from build123d import *

# Parameters (mm, degrees)
SKETCH1_R           = 7.5
BOSS_EXTRUDE2_DEPTH = 5
BOSS_EXTRUDE5_START = 2.5
SKETCH4_R           = 5
BOSS_EXTRUDE5_DEPTH = 5
BOSS_EXTRUDE6_START = -7.5
SKETCH4_2_R         = 5
BOSS_EXTRUDE6_DEPTH = 5
CIRPATTERN5_COUNT   = 3
CIRPATTERN5_ANGLE   = 240


with BuildPart() as part:
    # Sketch1 → Boss-Extrude2 (new body)
    with BuildSketch(Plane(origin=(0, 0, 0), x_dir=(1, 0, 0), z_dir=(0, 1, 0))):
        with BuildLine():
            Line((-15, 98.868599666), (-15, 128.868599666))
            Line((-15, 128.868599666), (15, 128.868599666))
            Line((15, 128.868599666), (15, 98.868599666))
            ThreePointArc((15, 98.868599666), (86.602540378, 50), (93.122718948, -36.443918776))
            Line((93.122718948, -36.443918776), (119.103481061, -51.443918776))
            Line((119.103481061, -51.443918776), (104.103481061, -77.42468089))
            Line((104.103481061, -77.42468089), (78.122718948, -62.42468089))
            ThreePointArc((78.122718948, -62.42468089), (0, -100), (-78.122718948, -62.42468089))
            Line((-78.122718948, -62.42468089), (-104.103481061, -77.42468089))
            Line((-104.103481061, -77.42468089), (-119.103481061, -51.443918776))
            Line((-119.103481061, -51.443918776), (-93.122718948, -36.443918776))
            ThreePointArc((-93.122718948, -36.443918776), (-86.602540378, 50), (-15, 98.868599666))
        make_face()
        with Locations(Location((0, 0, 0), (0, 0, 270))):
            Circle(SKETCH1_R, mode=Mode.SUBTRACT)
    extrude(amount=BOSS_EXTRUDE2_DEPTH)

    # Sketch4 → Boss-Extrude5 (add)
    with BuildSketch(Plane(origin=(0, 0, 0), x_dir=(0, 0, -1), z_dir=(1, 0, 0)).offset(BOSS_EXTRUDE5_START)):
        with BuildLine():
            Line((104.299170688, -17.902762311), (98.868599666, 0))
            Line((98.868599666, 0), (128.868599666, 0))
            Line((128.868599666, 0), (123.438028644, -17.902762311))
            ThreePointArc((123.438028644, -17.902762311), (113.868599666, -25), (104.299170688, -17.902762311))
        make_face()
        with Locations((113.868599666, -15)):
            Circle(SKETCH4_R, mode=Mode.SUBTRACT)
    boss_extrude5 = extrude(amount=BOSS_EXTRUDE5_DEPTH)

    # Sketch4_2 → Boss-Extrude6 (add)
    with BuildSketch(Plane(origin=(0, 0, 0), x_dir=(0, 0, -1), z_dir=(1, 0, 0)).offset(BOSS_EXTRUDE6_START)):
        with BuildLine():
            Line((104.299170688, -17.902762311), (98.868599666, 0))
            Line((98.868599666, 0), (128.868599666, 0))
            Line((128.868599666, 0), (123.438028644, -17.902762311))
            ThreePointArc((123.438028644, -17.902762311), (113.868599666, -25), (104.299170688, -17.902762311))
        make_face()
        with Locations((113.868599666, -15)):
            Circle(SKETCH4_2_R, mode=Mode.SUBTRACT)
    boss_extrude6 = extrude(amount=BOSS_EXTRUDE6_DEPTH)

    # CirPattern5: Boss-Extrude5, Boss-Extrude6 ×3 about axis
    cirpattern5_axis = Axis((0, 0, 0), (0, 1, 0))
    add([boss_extrude5.rotate(cirpattern5_axis, i * CIRPATTERN5_ANGLE / (CIRPATTERN5_COUNT - 1)) for i in range(1, CIRPATTERN5_COUNT)])
    add([boss_extrude6.rotate(cirpattern5_axis, i * CIRPATTERN5_ANGLE / (CIRPATTERN5_COUNT - 1)) for i in range(1, CIRPATTERN5_COUNT)])


solid = part.part
Design review of the part built by this model. Coordinates are the model's own, in mm. A direction names the side the tool comes from. Give positions to 0.01 mm unless a question says otherwise; leave off trailing zeros. Order: outer loops, then holes, each group sorted by start corner. A loop starts at its lowest first (then second) coordinate and runs counter-clockwise, first axis right, second up. Notation, with made-up numbers: (25.25, 55) - (52.25, 55) arc R29 ccw to (52.25, 80) - close; hole circle Ø10 at (-27.5, 83). An arc over 180 degrees is marked (long way). Write item = value, one per line. Start each with the question number.
Q1. Tool access review of faces 5 (the face through (102.54, -9.55, 50.54)), 6 (the face through (-7.5, -9.5, -114.1)), 7 (the face through (-106.295, 2.465, 44.049)), 8 (the face through (-95.04, -9.55, 63.53)): name each direction out of +Z, -Z, +X, -X, +Y, -Y from which nothing blocks a thin tool from reaching the whole face with its end or side.
Q2. We need section B-B on y = -3.75. State the section outline as (x, z) points, plus the area to 3 significant figures.
Q3. We need section C-C on x = 28. State the section outline as (y, z) points.
Q4. To check wall thickness, follow L1, parallel to X at y = 2.3, z = 0; L2, parallel to X at y = -7.25, z = -115.5; L3, parallel to X at y = 0.5, z = -100. State the ranges of each line that lie inside material, in increasing order. Write a range as from..to.
Q5. Clearance check with flat-ended pins moving along their axes: pin 1 Ø5.5 at (y, z) = (1.5, -116) entering from -X; pin 2 Ø12.5 at (y, z) = (-7.5, -121) entering from +X; pin 3 Ø11.5 at (y, z) = (-15, -113.87) entering from -X. State where each tip first meets the part, or that it passes through.
Q6. We need section D-D on z = -39. State the section outline as (x, y) points.
Q7. We need section A-A on z = 0. State the section outline as (x, y) points.
Q8. Mouldability with a two-part tool opening along Z and no side actions: class faces 1 (the face through (0.33, 2.465, -7.493)), 2 (the face through (105.13, -16.92, 54.88)), 3 (the face through (-5, -25, -114)), 4 (the face through (106.8, -8.83, 67.4)) as released by +Z, released by -Z, zero draft, split by the parting line, or undercut.
Working result:
q1.face_5 = -Z, +X, -Y
q1.face_6 = +Z, -Z, -X, -Y
q1.face_7 = -X, +Y, -Y
q1.face_8 = +Z, -Y
q2.outline = (-114.37, 57.37) - (-90.36, 43.51) - (-87.86, 47.84) - (-111.87, 61.7) - close; (-109.37, 66.03) - (-85.36, 52.17) - (-82.86, 56.5) - (-106.87, 70.36) - close; (-7.5, -127.73) - (-2.5, -127.73) - (-2.5, -100.01) - (-7.5, -100.01) - close; (2.5, -127.73) - (7.5, -127.73) - (7.5, -100.01) - (2.5, -100.01) - close; (82.86, 56.5) - (85.36, 52.17) - (109.37, 66.03) - (106.87, 70.36) - close; (87.86, 47.84) - (90.36, 43.51) - (114.37, 57.37) - (111.87, 61.7) - close
q2.area = 832 mm²
q3.outline = (0, -96) - (5, -96) - (5, 96) - (0, 96) - close
q4.L1 = -100..-7.5, 7.5..100
q4.L2 = -7.5..-2.5, 2.5..7.5
q4.L3 = -15..15
q5.pin_1 = -15
q5.pin_2 = 7.5
q5.pin_3 = -7.5
q6.outline = (-92.08, 0) - (92.08, 0) - (92.08, 5) - (-92.08, 5) - close
q7.outline = (-100, 0) - (-7.5, 0) - (-7.5, 5) - (-100, 5) - close; (7.5, 0) - (100, 0) - (100, 5) - (7.5, 5) - close
q8.face_1 = undercut
q8.face_2 = undercut
q8.face_3 = split by the parting line
q8.face_4 = released by +Z
